Design review of the part built by this model. Coordinates are the model's own, in mm. Face numbers are marked on the shaded views. A direction names the side the tool comes from. Coordinates: 2 decimals unless noted, no trailing zeros. Loops run counter-clockwise (first coordinate to the right, second up) from the corner with the lowest first, then second, coordinate; pieces in that order, holes last. Notation, with made-up numbers: M 1,-28 L 22,-28 A19 cw 22,-7 Z; hole C 53.5,82.25 d6. An arc over 180 degrees is marked long. Put each result on its own line as item: value. Start each with the question number.
(1) For probe 1 along Z at (x, y) = (-22, -8.5); probe 2 along X at (y, z) = (-3, 12.5); probe 3 along Y at (x, z) = (27.5, 2.15), list the stretches that pass through material, from the lowest coordinate up. Write a range as [from, to].
(2) Take a section at A-A, the plane x = 27.5. Give the boundary of the cut face in (y, z).
(3) Clearance check with flat-ended pins moving along their axes: pin 1 (7 mm diameter, centred on x = -30, y = -2, fed in from +Z); pin 2 (2 mm diameter, centred on y = 0.5, z = 13.5, fed in from +X); pin 3 (6 mm diameter, centred on y = 2, z = 9.5, fed in from -X). State where each tip first meets the part, or that it passes through.
(4) For the marked faces 1, 2 and 3, list the 3-axis set-ups (+Z, -Z, +X, -X, +Y, -Y) from which the entire face can be reached by the end or side of a thin tool; tool diameter is ignored.
(5) Take a section at B-B, the plane z = 10.75. Give the boundary of the cut face in (x, y), then the cut area to 3 significant figures.
(6) Take a section at C-C, the plane y = -15. Give the boundary of the cut face in (x, z), then the cut area to 3 significant figures.
(7) The part is to be moulded in two halves that separate along Y. For the marked faces 4, 5, 6 and 7, say which applies: +Y half, -Y half, draft (parallel to the pull), parting line (faces both ways), or undercut.
(8) Take a section at D-D, the plane x = -27.5. Give the boundary of the cut face in (y, z).
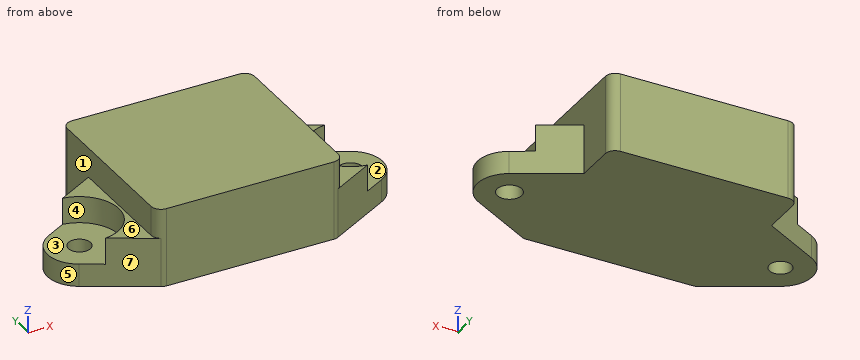
Autodesk Inventor part; units mm, degrees
ref_plane "XZ Plane" through (0, 0, 0) normal (0, 1, 0) x (-1, 0, 0)
sketch "Sketch1" plane through (0, 0, 0) normal (0, 0, 1) x (1, 0, 0)
  line L0 (-19, 16.7257) -> (19, 16.7257)
  line L1 (19, 16.7257) -> (19, -18.2743)
  line L2 (19, -18.2743) -> (-19, -18.2743)
  line L3 (-19, -18.2743) -> (-19, 16.7257)
  line L4 (0, 21.1891) -> (0, -25.1053) construction
  line L5 (31.0331, 0) -> (-23.8841, 0) construction
  point P0 (0, 0)
  dimension "d0" = 38
  dimension "d1" = 35
extrude "Extrusion1" add sketch "Sketch1" along normal blind 16
fillet "Fillet1" radius 2 4 edges at (19, 16.7257, 8) (19, -18.2743, 8) (-19, 16.7257, 8) (-19, -18.2743, 8)
sketch "Sketch2" plane through (0, 0, 0) normal (0, 0, 1) x (1, 0, 0)
  line L0 (-19, 14.7257) -> (-19, -16.2743)
  line L1 (17, 16.7257) -> (-17, 16.7257)
  line L2 (19, -16.2743) -> (19, 14.7257)
  line L3 (-17, -18.2743) -> (17, -18.2743)
  arc A0 (30.6631, -10.9527) -> (30.6631, 0.4041) centre (27.5, -5.2743) ccw
  line L4 (30.6631, 0.4041) -> (19, 6.901)
  line L5 (-28.9465, 0) -> (40.6791, 0)
  line L6 (0, 23.9357) -> (0, -26.5345)
  arc A1 (17, -18.2743) -> (19, -16.2743) centre (17, -16.2743) ccw
  line L7 (30.6631, -10.9527) -> (17.9733, -18.0215)
  line L8 (19, 6.901) -> (19, -16.2743)
  arc A2 (17.9733, -18.0215) -> (19, -16.2743) centre (17, -16.2743) ccw
  point P0 (0, 0)
  dimension "d5" = 27.5
  dimension "d6" = 13
  dimension "d7" = 6.5
  dimension "d8" = 29.12
  dimension "d9" = 29.12
extrude "Extrusion2" add sketch "Sketch2" along normal blind 10 contours L2 L5 A0 L7 A1 | L2 L4 A0 L5
sketch "Sketch3" plane through (0, 0, 10) normal (0, 0, 1) x (1, 0, 0)
  arc A0 (30.6631, -10.9527) -> (30.6631, 0.4041) centre (27.5, -5.2743) ccw construction
  point P0 (0, 0)
hole "Hole1" at (27.5, -5.2743, 10) direction (0, 0, -1) diameter 16 depth 5.4
mirror "Mirror1" about plane through (0, 0, 0) normal (1, 0, 0) of "Extrusion2", "Hole1"
sketch "Sketch4" plane through (27.5, -5.2743, 4.6) normal (0, 0, 1) x (1, 0, 0)
  arc A0 (3.1631, -5.6784) -> (3.1631, 5.6784) centre (0, 0) ccw construction
  line L0 (-58.1631, 5.6784) -> (-54.0889, 7.9479) construction
  arc A1 (-58.1631, 5.6784) -> (-58.1631, -5.6784) centre (-55, 0) ccw construction
  line L1 (-54.0889, -7.9479) -> (-58.1631, -5.6784) construction
  arc A2 (-54.0889, -7.9479) -> (-54.0889, 7.9479) centre (-55, 0) ccw construction
  point P0 (-27.5, 5.2743)
hole "Hole2" at (27.5, -5.2743, 4.6) direction (0, 0, -1) diameter 5 end through all
sketch "Sketch5" plane through (-27.5, -5.2743, 4.6) normal (0, 0, 1) x (1, 0, 0)
  arc A0 (-3.1631, 5.6784) -> (-3.1631, -5.6784) centre (0, 0) ccw construction
  point P0 (27.5, 5.2743)
hole "Hole3" at (-27.5, -5.2743, 4.6) direction (0, 0, -1) diameter 4.5 end through all
equation "\"d9\" = d8"
properties part number "TPS"
Computed values:
1. probe 1: z = [0, 4.6]
1. probe 2: x = [-19, 19]
1. probe 3: y = [-12.71, -7.77], [-2.77, 2.17]
2. outline: M -12.71,0 L -7.77,0 L -7.77,4.6 L -12.71,4.6 Z; M -2.77,0 L 2.17,0 L 2.17,4.6 L -2.77,4.6 Z
3. pin 1: stops at z = 4.6
3. pin 2: stops at x = 19
3. pin 3: stops at x = -26.59
4. face 1: +Z, -X, +Y
4. face 2: +Z, +X
4. face 3: +Z, -X
5. outline: M -19,-16.27 A2 ccw -17,-18.27 L 17,-18.27 A2 ccw 19,-16.27 L 19,14.73 A2 ccw 17,16.73 L -17,16.73 A2 ccw -19,14.73 Z
5. area: 1,330 mm^2
6. outline: M -23.4,0 L 23.4,0 L 23.4,10 L 19,10 L 19,16 L -19,16 L -19,10 L -23.4,10 Z
6. area: 696 mm^2
7. face 4: undercut
7. face 5: parting line
7. face 6: draft
7. face 7: -Y half
8. outline: M -12.71,0 L -7.52,0 L -7.52,4.6 L -12.71,4.6 Z; M -3.02,0 L 2.17,0 L 2.17,4.6 L -3.02,4.6 Z
